Model file for the job. Use its own axes, mm. A direction names the side the tool comes from. Coordinates: 2 decimals unless noted, no trailing zeros. Write each loop counter-clockwise with the first axis right and the second up, starting at its lowest first coordinate (ties: lowest second). Pieces come first, ordered by that corner, then holes. Notation, with made-up numbers: M 27,30 L 77,30 A12 cw 77,39 Z; hole C 32.25,-6 d10. An arc over 180 degrees is marked long. Put each result on its own line as item: value. Start each with the question number.
Q1. Cut at B-B (y = 11.5). Write the cut outline in (x, z).
Q2. Drop a flat-ended pin along its axis: pin 1 (1.3 mm diameter, centred on x = 20.5, z = -35.5, fed in from +Y). Give the stop position or say it passes through.
Q3. Pull direction X, two halves, no side cores. Call faces 1 (the flat face through (1, 16.256, -45)), 2 (the flat face through (25.019, 8, -45)), 3 (the flat face through (12.978, 10, -45)): pulls with the +X half, pulls with the -X half, needs draft (parallel to the pull), parting line crosses it, or undercut.
Q4. Which spindle directions (+Z, -Z, +X, -X, +Y, -Y) get a long thin tool onto all of the face, cutting with end or side? Do faces 4 (the flat face through (12, 6, -92.202)), 5 (the flat face through (9, 3.302, -45)). Say none if no direction does.
Q5. Cut at A-A (z = -78.74). Write the cut outline in (x, y).
Q6. Drill centre lines: line 1 along X through (y, z) = (10.75, -30); line 2 along X through (y, z) = (1.4, -78.74); line 3 along Y through (x, z) = (21.5, -69). Where is each one in solid material? Low to high.
```python
from build123d import *

# Parameters (mm, degrees)
EXTRUDE1_DEPTH            = 92.202
F_4_40_TAPPED_HOLE1_D     = 2.2606
F_4_40_TAPPED_HOLE1_DEPTH = 7.5946
F_4_40_TAPPED_HOLE1_TIP   = 0.679152758


with BuildPart() as part:
    # Sketch1 → Extrude1 (new body)
    with BuildSketch(Plane.XY):
        Polygon((0, 0), (25.019, 0), (25.019, 16.256), (23.3934, 16.256), (23.3934, 3.302), (19.013003595, 3.302), (19.013003595, 16.256), (17.387403595, 16.256), (17.387403595, 3.302), (12.97763135, 3.302), (12.97763135, 16.256), (11.35203135, 16.256), (11.35203135, 3.302), (7.190288103, 3.302), (7.190288103, 16.256), (5.564688103, 16.256), (5.564688103, 3.302), (1.6256, 3.302), (1.6256, 16.256), (0, 16.256), align=None)
    extrude(amount=-EXTRUDE1_DEPTH)

    # #4-40 Tapped Hole1
    with Locations(Plane.XZ):
        with Locations((9.525, -25.4), (9.525, -78.74)):
            Hole(F_4_40_TAPPED_HOLE1_D / 2, depth=F_4_40_TAPPED_HOLE1_DEPTH)
            with Locations((0, 0, -(F_4_40_TAPPED_HOLE1_DEPTH + F_4_40_TAPPED_HOLE1_TIP / 2))):  # 118° drill point
                Cone(0, F_4_40_TAPPED_HOLE1_D / 2, F_4_40_TAPPED_HOLE1_TIP, mode=Mode.SUBTRACT)


solid = part.part
```
Computed values:
1. outline: M 0,-92.2 L 1.63,-92.2 L 1.63,0 L 0,0 Z; M 5.56,-92.2 L 7.19,-92.2 L 7.19,0 L 5.56,0 Z; M 11.35,-92.2 L 12.98,-92.2 L 12.98,0 L 11.35,0 Z; M 17.39,-92.2 L 19.01,-92.2 L 19.01,0 L 17.39,0 Z; M 23.39,-92.2 L 25.02,-92.2 L 25.02,0 L 23.39,0 Z
2. pin 1: y = 3.3
3. face 1: needs draft
3. face 2: pulls with the +X half
3. face 3: undercut
4. face 4: -Z, +X, -X, +Y, -Y
4. face 5: +Z, -Z, +Y
5. outline: M 0,0 L 8.39,0 L 8.39,3.3 L 7.19,3.3 L 7.19,16.26 L 5.56,16.26 L 5.56,3.3 L 1.63,3.3 L 1.63,16.26 L 0,16.26 Z; M 10.66,0 L 25.02,0 L 25.02,16.26 L 23.39,16.26 L 23.39,3.3 L 19.01,3.3 L 19.01,16.26 L 17.39,16.26 L 17.39,3.3 L 12.98,3.3 L 12.98,16.26 L 11.35,16.26 L 11.35,3.3 L 10.66,3.3 Z
6. line 1: 0 to 1.63, 5.56 to 7.19, 11.35 to 12.98, 17.39 to 19.01, 23.39 to 25.02
6. line 2: 0 to 8.39, 10.66 to 25.02
6. line 3: 0 to 3.3
